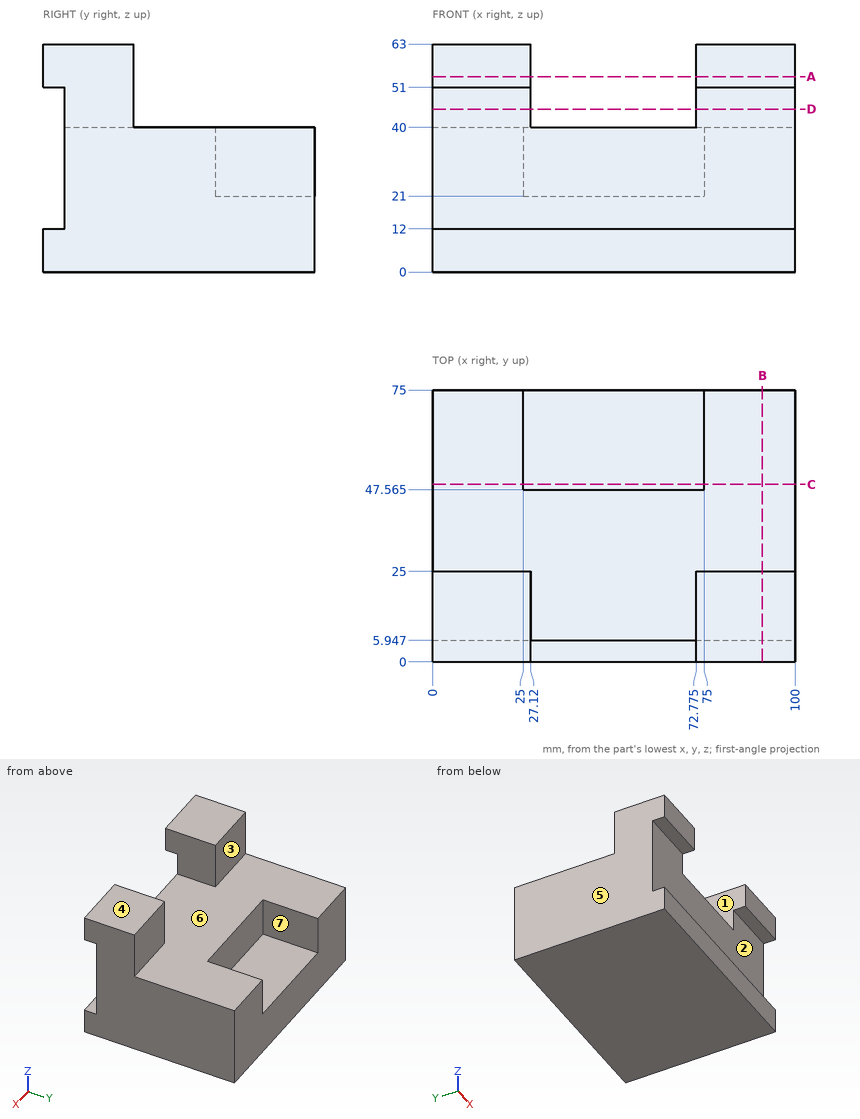
Design review of the part shown in the three views and the two pictorial views. Dimensions are in mm from the part's minimum x, y and z. A direction names the side the tool comes from. Coordinates: 2 decimals unless noted, no trailing zeros. Write each loop counter-clockwise with the first axis right and the second up, starting at its lowest first coordinate (ties: lowest second). Pieces come first, ordered by that corner, then holes.
(1) Tool access review of the marked faces 1, 2 and 3: name each direction out of +Z, -Z, +X, -X, +Y, -Y from which nothing blocks a thin tool from reaching the whole face with its end or side.
(2) Add section C-C on y = 49. Give the boundary of the cut face in (x, z).
(3) For pin 1 Ø22 at (x, y) = (54, 57) entering from +Z; pin 2 Ø7 at (x, z) = (20, 53) entering from +Y; pin 3 Ø5.5 at (y, z) = (61, 34) entering from -X; pin 4 Ø6.5 at (x, y) = (42, 2.5) entering from +Z, all flat-tipped, find the tip position at first contact; note any pin that passes through.
(4) Wall thickness on probe 1 along X at (y, z) = (48.5, 27); probe 2 along X at (y, z) = (22, 51) (1 decimal); probe 3 along Z at (x, y) = (89, 44.5): over which ranges is each line inside the solid? List them lowest first.
(5) Add section D-D on z = 45. Give the boundary of the cut face in (x, y) (1 decimal), then the cut area to 3 significant figures.
(6) The part is to be moulded in two halves that separate along X. For the marked faces 4, 5, 6 and 7, say which applies: +X half, -X half, draft (parallel to the pull), parting line (faces both ways), or undercut.
(7) Add section A-A on z = 54. Give the boundary of the cut face in (x, y) (1 decimal).
(8) Add section B-B on x = 91. Give the boundary of the cut face in (y, z).
Answer sheet:
1. face 1: +Z, +Y, -Y
1. face 2: +X, -X, -Y
1. face 3: +Z, +X, -X, +Y
2. outline: (0, 0) - (100, 0) - (100, 40) - (75, 40) - (75, 21) - (25, 21) - (25, 40) - (0, 40) - close
3. pin 1: stops at z = 40
3. pin 2: stops at y = 25
3. pin 3: stops at x = 0
3. pin 4: stops at z = 12
4. probe 1: x = 0 to 25, 75 to 100
4. probe 2: x = 0 to 27.1, 72.8 to 100
4. probe 3: z = 0 to 40
5. outline: (0, 5.9) - (27.1, 5.9) - (27.1, 25) - (0, 25) - close; (72.8, 5.9) - (100, 5.9) - (100, 25) - (72.8, 25) - close
5. area: 1,040 mm2
6. face 4: draft
6. face 5: -X half
6. face 6: undercut
6. face 7: undercut
7. outline: (0, 0) - (27.1, 0) - (27.1, 25) - (0, 25) - close; (72.8, 0) - (100, 0) - (100, 25) - (72.8, 25) - close
8. outline: (0, 0) - (75, 0) - (75, 40) - (25, 40) - (25, 63) - (0, 63) - (0, 51) - (5.95, 51) - (5.95, 12) - (0, 12) - close
